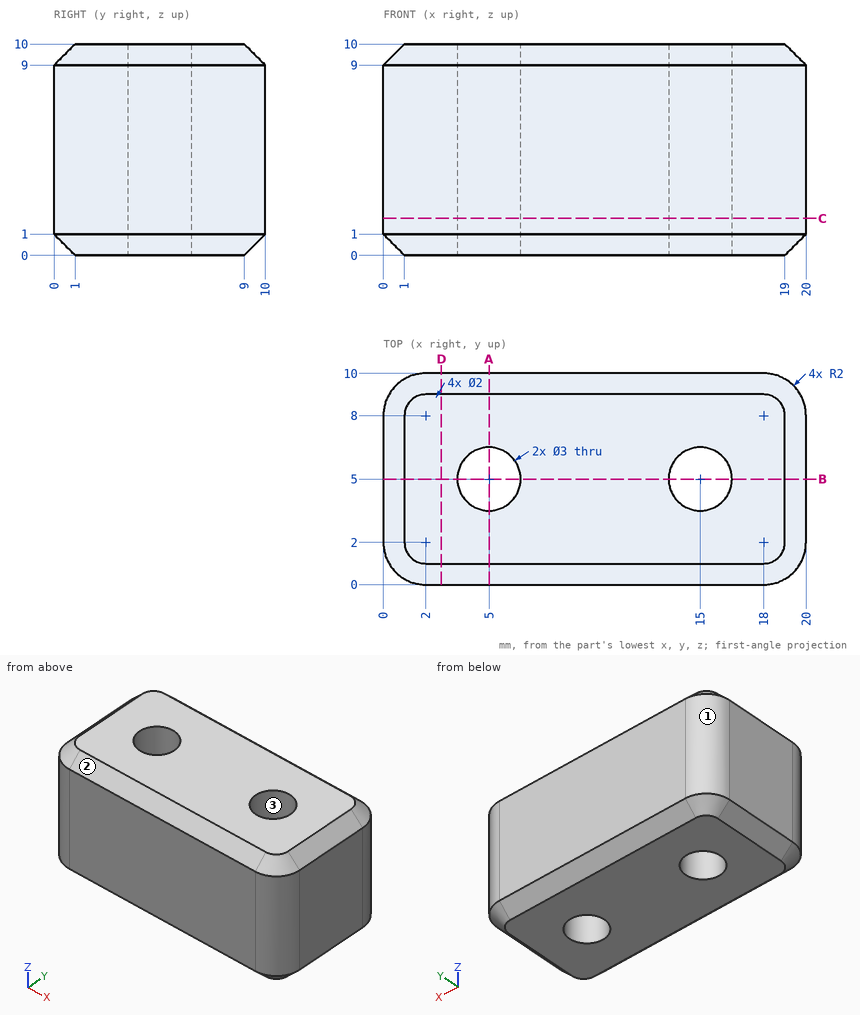
Can you work these out from the drawing? Everything is in mm from the part's minimum corner. Coordinates: 2 decimals unless noted, no trailing zeros. Order: outer loops, then holes, each group sorted by start corner. A loop starts at its lowest first (then second) coordinate and runs counter-clockwise, first axis right, second up. Notation, with made-up numbers: (-26.75, -18) -> (-20.75, -18) arc R22 cw to (-20.75, 12) -> close; hole circle Ø4 at (-20.75, -17). An arc over 180 degrees is marked (long way). Use one line per item in the form item = value.
Q1. Imagine slicing it at D-D, the plane x = 2.75. List the corners of the cut face in (y, z) for me, then the cut area to 3 significant figures.
From the geometry:
outline = (0, 1) -> (1, 0) -> (9, 0) -> (10, 1) -> (10, 9) -> (9, 10) -> (1, 10) -> (0, 9) -> close
area = 98.0 mm²
Q2. Imagine slicing it at B-B, the plane y = 5. List the corners of the cut face in (x, z) for me.
From the geometry:
outline = (0, 1) -> (1, 0) -> (3.5, 0) -> (3.5, 10) -> (1, 10) -> (0, 9) -> close; (6.5, 0) -> (13.5, 0) -> (13.5, 10) -> (6.5, 10) -> close; (16.5, 0) -> (19, 0) -> (20, 1) -> (20, 9) -> (19, 10) -> (16.5, 10) -> close
Q3. I need wall thicknesses on L1, parallel to X at y = 6.25, z = 2.75; L2, parallel to Y at x = 5, z = 3.25; L3, parallel to X at y = 4.75, z = 5.5. Which ranges of each line are inside material? Lowest first, please.
From the geometry:
L1 = 0 to 4.17, 5.83 to 14.17, 15.83 to 20
L2 = 0 to 3.5, 6.5 to 10
L3 = 0 to 3.52, 6.48 to 13.52, 16.48 to 20
Q4. Imagine slicing it at A-A, the plane x = 5. List the corners of the cut face in (y, z) for me, then the cut area to 3 significant figures.
From the geometry:
outline = (0, 1) -> (1, 0) -> (3.5, 0) -> (3.5, 10) -> (1, 10) -> (0, 9) -> close; (6.5, 0) -> (9, 0) -> (10, 1) -> (10, 9) -> (9, 10) -> (6.5, 10) -> close
area = 68.0 mm²
Q5. Will this pin go through, and if not, where does the flat tip stop? P1, Ø5, axis at y = 6, z = 9, coming from the -X side.
From the geometry:
P1 = 0
Q6. Imagine slicing it at C-C, the plane z = 1.75. List the corners of the cut face in (x, y) for me.
From the geometry:
outline = (0, 2) arc R2 ccw to (2, 0) -> (18, 0) arc R2 ccw to (20, 2) -> (20, 8) arc R2 ccw to (18, 10) -> (2, 10) arc R2 ccw to (0, 8) -> close; hole circle Ø3 at (5, 5); hole circle Ø3 at (15, 5)
Q7. We'd pull the mould along X, two halves only. Please class the marked faces 1, 2 and 3: released by +X, released by -X, zero draft, split by the parting line, or undercut.
From the geometry:
face_1 = released by -X
face_2 = zero draft
face_3 = undercut
